Build history of the part. All positions in model axes, mm. Face numbers are marked on the shaded views. A direction names the side the tool comes from. Give positions to 0.01 mm unless a question says otherwise; leave off trailing zeros. Loops run counter-clockwise (first coordinate to the right, second up) from the corner with the lowest first, then second, coordinate; pieces in that order, holes last. Notation, with made-up numbers: (11.5, 1.5) - (65.5, 1.5) arc R7 cw to (65.5, 6.5) - close; hole circle Ø4 at (40.5, 57). An arc over 180 degrees is marked (long way). Return JSON: item names as keys, results as strings. Group by question number.
1) Mould opens along Y. For the marked faces 1, 2 and 3 say: released by +Y, released by -Y, zero draft, split by the parting line, or undercut.
2) Slice it at A-A (z = 8). List the corners of the cut face in (x, y), and give its area (3 significant figures).
3) Slice it at B-B (x = 11.5). List the corners of the cut face in (y, z), and give its area (3 significant figures).
4) Drill centre lines: probe 1 along Z at (x, y) = (34, -16); probe 2 along Y at (x, z) = (103, 3.75); probe 3 along X at (y, z) = (-11, 35.5). Where is each one in solid material? Low to high. Write a range as from..to.
5) Slice it at C-C (z = 46). List the corners of the cut face in (x, y).
6) Drop flat-ended pins along their axis: pin 1 (5 mm diameter, centred on x = 26.5, y = -25.5, fed in from +Z); pin 2 (16 mm diameter, centred on y = -16.5, z = 31, fed in from -X); pin 3 (16 mm diameter, centred on x = 62, y = -18.5, fed in from -Z). Give the stop position or say it passes through.
7) Slice it at D-D (y = -13). Count the separate pieces of the cut face and the enclosed holes in it, and give its area (3 significant figures).
8) 3-axis set-ups, long thin cutter, end or side, ignore diameter. For the marked faces 4, 5 and 6: which of +Z, -Z, +X, -X, +Y, -Y reach the whole face in a straight line?
```python
from build123d import *

# Parameters (mm, degrees)
F0_W      = 113
F0_H      = 64
F1_DEPTH  = 32
F2_W      = 20
F2_H      = 51
F2_W_2    = 35
F2_H_2    = 34
F2_H_3    = 17
F3_DEPTH  = 32.001
F5_DEPTH  = 25
F7_DEPTH  = 93.001
F8_R      = 6.5
F9_DEPTH  = 93.001
F11_R     = 5.5
F10_R     = 5.5
F12_DEPTH = 13.001


with BuildPart() as f1:
    # F0 (on Front) → F1 (new body)
    with BuildSketch(Plane.XZ):
        with Locations((56.5, 32)):
            Rectangle(F0_W, F0_H)
    extrude(amount=F1_DEPTH)

    # F2 (on face) → F3 (cut, through all)
    with BuildSketch(Plane.XZ.offset(32)):
        with Locations((10, 38.5)):
            Rectangle(F2_W, F2_H)
        with Locations((56.5, 47)):
            Rectangle(F2_W_2, F2_H_2)
        with Locations((56.5, 8.5)):
            Rectangle(F2_W_2, F2_H_3)
        with Locations((103, 38.5)):
            Rectangle(F2_W, F2_H)
    extrude(amount=-F3_DEPTH, mode=Mode.SUBTRACT)

    # F4 (on face) → F5 (cut)
    with BuildSketch(Plane.XY.offset(13)):
        Polygon((103, -32), (113, -32), (113, -22), align=None)
        Polygon((0, -22), (0, -32), (10, -32), align=None)
    extrude(amount=-F5_DEPTH, mode=Mode.SUBTRACT)

    # F6 (on face) → F7 (cut, through all)
    with BuildSketch(Plane.YZ.offset(93)):
        with BuildLine():
            ThreePointArc((-32, 60.2490309932), (-24.2168997878, 63.0497155178), (-16, 64))
            Line((-16, 64), (-32, 64))
            Line((-32, 64), (-32, 60.2490309932))
        make_face()
        with BuildLine():
            ThreePointArc((-16, 64), (-7.7831002122, 63.0497155178), (0, 60.2490309932))
            Line((0, 60.2490309932), (0, 64))
            Line((0, 64), (-16, 64))
        make_face()
    extrude(amount=-F7_DEPTH, mode=Mode.SUBTRACT)

    # F8 (on face) → F9 (cut, through all)
    with BuildSketch(Plane.YZ.offset(93)):
        with Locations((-16, 46)):
            Circle(F8_R)
    extrude(amount=-F9_DEPTH, mode=Mode.SUBTRACT)

    # F11 (on face) + F10 (on face) → F12 (cut, through all)
    with BuildSketch(Plane.XY.offset(13)):
        with Locations((103, -13)):
            Circle(F11_R)
    with BuildSketch(Plane.XY.offset(13)):
        with Locations((10, -13)):
            Circle(F10_R)
    extrude(amount=-F12_DEPTH, mode=Mode.SUBTRACT)


solid = f1.part
```
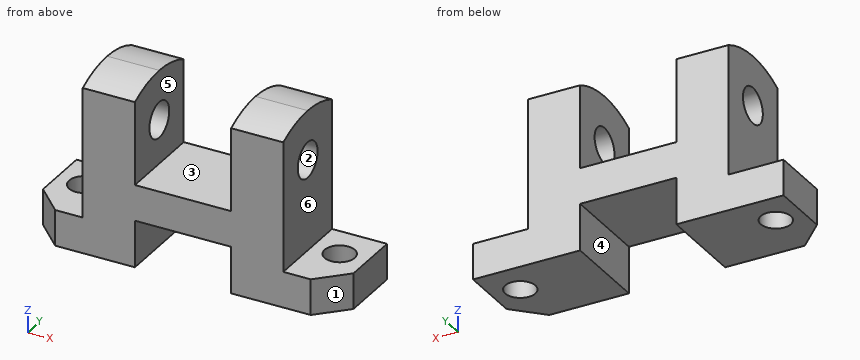
Results:
{
 "1": {"face 1": "released by -Y", "face 2": "undercut", "face 3": "zero draft"},
 "2": {"outline": "(0, -22) - (10, -32) - (39, -32) - (39, 0) - (0, 0) - close; (74, -32) - (103, -32) - (113, -22) - (113, 0) - (74, 0) - close; hole circle Ø11 at (10, -13); hole circle Ø11 at (103, -13)", "area": "2,210 mm2"},
 "3": {"outline": "(-32, 0) - (-18.29, 0) - (-18.29, 13) - (-32, 13) - close; (-7.71, 0) - (0, 0) - (0, 13) - (-7.71, 13) - close", "area": "278 mm2"},
 "4": {"probe 1": "0..39.5, 52.5..64", "probe 2": "-32..-18.5, -7.5..0", "probe 3": "20..39, 74..93"},
 "5": {"outline": "(20, -32) - (39, -32) - (39, -22.5) - (20, -22.5) - close; (20, -9.5) - (39, -9.5) - (39, 0) - (20, 0) - close; (74, -32) - (93, -32) - (93, -22.5) - (74, -22.5) - close; (74, -9.5) - (93, -9.5) - (93, 0) - (74, 0) - close"},
 "6": {"pin 1": "z = 63.31", "pin 2": "x = 20", "pin 3": "z = 17"},
 "7": {"separate pieces": "5", "enclosed holes": "0", "area": "2,680 mm2"},
 "8": {"face 4": "-Z, +Y, -Y", "face 5": "+Z, +Y, -Y", "face 6": "+Z, +X, +Y, -Y"}
}
